```python
from build123d import *

# Parameters (mm, degrees)
SKETCH1_W                  = 113
SKETCH1_H                  = 107
MAIN_BODY_BACK_PLATE_DEPTH = 5
HEIGHT_ADJUST_DEPTH        = 20
SKETCH4_W                  = 23
SKETCH4_H                  = 10
SKETCH4_H_2                = 9.5
HOLE_POSTITIONS_DEPTH      = 40
SKETCH5_R                  = 2
SCREW_HOLES_DEPTH          = 10.59530888
FILLET1_R                  = 4
SKETCH6_W                  = 9.5
SKETCH6_H                  = 27
CUT_EXTRUDE1_DEPTH         = 10
FILLET2_R                  = 3.5


with BuildPart() as part:
    # Sketch1 → Main Body Back Plate (new body)
    with BuildSketch(Plane(origin=(0, 0, 0), x_dir=(1, 0, 0), z_dir=(0, 1, 0))):
        Rectangle(SKETCH1_W, SKETCH1_H)
    extrude(amount=MAIN_BODY_BACK_PLATE_DEPTH)

    # Sketch3 → Height Adjust (add, symmetric)
    with BuildSketch(Plane.ZY):
        Polygon((33.5, 0), (33.5, -4.59530888), (53.5, 0), align=None)
    extrude(amount=HEIGHT_ADJUST_DEPTH, both=True)

    # Sketch4 → Hole Postitions (cut)
    with BuildSketch(Plane(origin=(0, 5, 0), x_dir=(1, 0, 0), z_dir=(0, 1, 0))):
        with Locations((-14.5, 33)):
            Rectangle(SKETCH4_W, SKETCH4_H)
        with Locations((14.75, 33.25)):
            Rectangle(SKETCH4_W, SKETCH4_H_2)
    extrude(amount=-HOLE_POSTITIONS_DEPTH, mode=Mode.SUBTRACT)

    # Sketch5 → Screw Holes (cut, through all)
    with BuildSketch(Plane(origin=(0, 5, 0), x_dir=(1, 0, 0), z_dir=(0, 1, 0))):
        with Locations((-51.5, 48.5)):
            Circle(SKETCH5_R)
        with Locations((-51.5, -48.5)):
            Circle(SKETCH5_R)
        with Locations((51.5, -48.5)):
            Circle(SKETCH5_R)
        with Locations((51.5, 48.5)):
            Circle(SKETCH5_R)
    extrude(amount=-SCREW_HOLES_DEPTH, mode=Mode.SUBTRACT)

    # Fillet1
    fillet1_edges = [part.edges().sort_by_distance(p)[0] for p in [
        (56.5, 2.5, 53.5),
        (-56.5, 2.5, 53.5),
        (-56.5, 2.5, -53.5),
        (56.5, 2.5, -53.5),
    ]]
    fillet(fillet1_edges, radius=FILLET1_R)

    # Sketch6 → Cut-Extrude1 (cut)
    with BuildSketch(Plane.XZ):
        with Locations((-51.75, -8.75)):
            Rectangle(SKETCH6_W, SKETCH6_H)
    extrude(amount=-CUT_EXTRUDE1_DEPTH, mode=Mode.SUBTRACT)

    # Fillet2
    fillet2_edges = [part.edges().sort_by_distance(p)[0] for p in [
        (-56.5, 2.5, -22.25),
        (-56.5, 2.5, 4.75),
        (-47, 2.5, 4.75),
        (-47, 2.5, -22.25),
    ]]
    fillet(fillet2_edges, radius=FILLET2_R)


solid = part.part
```
Check sheet for the modelled part. Datum: model origin and axes. Units: mm. A direction names the side the tool comes from. Give positions to 0.01 mm unless a question says otherwise; leave off trailing zeros. Write each loop counter-clockwise with the first axis right and the second up, starting at its lowest first coordinate (ties: lowest second). Pieces come first, ordered by that corner, then holes. Notation, with made-up numbers: (-11.5, -35.75) -> (16.5, -35.75) arc R8 ccw to (16.5, -21.75) -> close; hole circle Ø7 at (10, 13). An arc over 180 degrees is marked (long way). Use CSV: the item, a comma, the result in double quotes. Start each with the question number.
Q1. Cross-section at B-B on z = 16. Enter the section's corners in (x, y).
Q2. Cross-section at C-C on x = -43.5. Enter the section's corners in (y, z).
Q3. Tool access check on faces 1 (the flat face through (3.25, 3, -33)), 2 (the flat face through (0, -2, 33.5)), 3 (the cylindrical face through (-55.4, 2.5, -23.2)). Record the directions out of +Z, -Z, +X, -X, +Y, -Y that give a thin tool (end or side, any length) a straight path to the whole face; none if there is none.
Q4. Scan lines: line 1 along Z through (x, y) = (51.5, 1.05); line 2 along X through (y, z) = (1.4, 48.5); line 3 along Z through (x, y) = (-51.5, 3.4). Record each from-to range of solid material in increasing order.
Q5. Cross-section at A-A on x = -4.5. Enter the section's corners in (y, z).
Q6. Release check for a two-part mould opening along Z. For faces 4 (the flat face through (-0.28, -2.33, 43.36)), 5 (the flat face through (-52, 2, 4.75)), 6 (the cylindrical face through (55.297, 2.535, -52.359)) record: +Z half, -Z half, draft (parallel to the pull), parting line (faces both ways), or undercut.
Q7. Depth check by flat-ended pin: P1, Ø1.5, axis at y = 3, z = -8.5, coming from the -X side; P2, Ø3, axis at x = -30, y = -3, coming from the +Z side; P3, Ø6.5, axis at x = 51.5, z = 48.5, coming from the -Y side; P4, Ø2.5, axis at x = -8, y = -1.5, coming from the -Z side. Enter the tip coordinate at first touch or a pass-through.
Working result:
1,outline,"(-56.5, 0) -> (56.5, 0) -> (56.5, 5) -> (-56.5, 5) -> close"
2,outline,"(0, -53.5) -> (5, -53.5) -> (5, 53.5) -> (0, 53.5) -> close"
3,face 1,"+Y, -Y"
3,face 2,"-Z, +X, -X, -Y"
3,face 3,"-X, +Y, -Y"
4,line 1,"z = -53.5 to -50.5, -46.5 to 46.5, 50.5 to 53.5"
4,line 2,"x = -56.5 to -53.5, -49.5 to 49.5, 53.5 to 56.5"
4,line 3,"z = -53.5 to -50.5, -46.5 to -22.25, 4.75 to 46.5, 50.5 to 53.5"
5,outline,"(-4.6, 33.5) -> (0, 33.5) -> (0, -28) -> (5, -28) -> (5, 53.5) -> (0, 53.5) -> close; (0, -53.5) -> (5, -53.5) -> (5, -38) -> (0, -38) -> close"
6,face 4,"+Z half"
6,face 5,"undercut"
6,face 6,"-Z half"
7,P1,"stops at x = -47"
7,P2,"passes through"
7,P3,"stops at y = 0"
7,P4,"stops at z = 33.5"
